Could you check a few things on this model? Use its own coordinates, in mm. A direction names the side the tool comes from. Round coordinates to 2 decimals unless told otherwise and drop trailing zeros. Loops run counter-clockwise (first coordinate to the right, second up) from the corner with the lowest first, then second, coordinate; pieces in that order, holes last. Notation, with made-up numbers: M -23.5,81 L -2.5,81 A19 ccw -2.5,94 Z; hole C 4,6 d1. An arc over 180 degrees is marked long. One line per item, written item: value. Start each with the question number.
Q1. Imagine slicing it at C-C (y = -10). Please give me the cut outline in (x, z) (3 decimals).
Q2. Which directions (+Z, -Z, +X, -X, +Y, -Y) give clear straight access to the entire face, cutting with the end or side of a thin tool? Please do faces 1 (the face through (4.639, -1.331, 5.637)), 2 (the face through (6.05, -1, 0)), 3 (the face through (-4.639, -1.331, -5.637)), 4 (the face through (-5, -2.7, 6)), 5 (the face through (-6.4, 0, 0)).
Q3. Imagine slicing it at D-D (x = 9.5). Please give me the cut outline in (y, z) (3 decimals).
Q4. Imagine slicing it at B-B (z = 0). Please give me the cut outline in (x, y).
Q5. Thinking about a two-plate mould opening in Y: for faces 6 (the face through (0, -23, 0)), 7 (the face through (10.8, -11, 0)), 8 (the face through (4.68, -1.33, -5.6)), which applies, released by +Y, released by -Y, zero draft, split by the parting line, or undercut?
Q6. I'm going to push flat-ended pins straight in: pin 1 Ø6 at (x, y) = (1.5, 3) entering from -Z; pin 2 Ø1.5 at (y, z) = (10, -3.5) entering from -X; pin 3 Ø6 at (y, z) = (-15, -3.5) entering from -X. Where does each tip first touch, or does it pass through?
Q7. Please list where these lines run through material, in increasing order: line 1 along Y through (x, z) = (6.75, 1.75); line 2 along Z through (x, y) = (0, -0.5); line 3 along X through (y, z) = (-5, -2.5).
Q8. Imagine slicing it at A-A (x = 0). Please give me the cut outline in (y, z).
Autodesk Inventor part; units mm, degrees
ref_plane "YZ Plane" through (0, 0, 0) normal (1, 0, 0) x (0, 1, 0)
ref_plane "XZ Plane" through (0, 0, 0) normal (0, 1, 0) x (-1, 0, 0)
ref_plane "XY Plane" through (0, 0, 0) normal (0, 0, 1) x (1, 0, 0)
sketch "Sketch1" plane through (0, 0, 0) normal (0, 1, 0) x (-1, 0, 0)
  circle A0 centre (0, 0) radius 7.9
  dimension "d0" = 15.8
extrude "Extrusion1" add sketch "Sketch1" along normal blind 18.9
sketch "Sketch2" plane through (0, 18.9, 0) normal (0, 1, 0) x (1, 0, 0)
  circle A0 centre (0, 0) radius 8.8
  dimension "d3" = 17.6
extrude "Extrusion2" add sketch "Sketch2" along normal blind 1.8
chamfer "Chamfer1" distance 1.5 angle 45 1 edges at (-8.8, 20.7, 0)
sketch "Sketch3" plane through (0, 0, 0) normal (0, -1, 0) x (1, 0, 0)
  line L0 (6.05, 6.7) -> (-6.05, 6.7)
  line L1 (-6.05, 6.7) -> (-6.05, -6.7)
  line L2 (-6.05, -6.7) -> (6.05, -6.7)
  line L3 (6.05, -6.7) -> (6.05, 6.7)
  line L4 (6.05, 6.7) -> (-6.05, -6.7) construction
  line L5 (-6.05, 6.7) -> (6.05, -6.7) construction
  point P0 (0, 0)
  dimension "d9" = 12.1
  dimension "d10" = 13.4
extrude "Extrusion3" add sketch "Sketch3" along normal blind 23
sketch "Sketch4" plane through (0, -23, 0) normal (0, -1, 0) x (1, 0, 0)
  line L0 (6.05, -6.7) -> (6.05, 6.7)
  line L1 (10.8, 4.525) -> (1.3, 4.525)
  line L2 (1.3, 4.525) -> (1.3, -4.525)
  line L3 (1.3, -4.525) -> (10.8, -4.525)
  line L4 (10.8, -4.525) -> (10.8, 4.525)
  line L5 (6.05, 5.0801) -> (6.05, -5.0801)
  line L6 (10.8, 4.525) -> (1.3, -4.525) construction
  line L7 (1.3, 4.525) -> (10.8, -4.525) construction
  point P0 (0, 0)
  point P1 (6.05, 0)
  dimension "d13" = 9.5
  dimension "d14" = 9.05
extrude "Extrusion4" add sketch "Sketch4" against normal blind 20.3
sketch "Sketch5" plane through (10.8, -23, 4.525) normal (1, 0, 0) x (0, 0, -1)
  line L0 (9.05, 0) -> (0, 0)
  line L1 (9.05, 4.67) -> (0, 4.67)
  line L2 (0, 4.67) -> (9.05, 4.67)
  line L3 (9.05, 4.67) -> (9.05, 0)
  line L4 (9.05, 0) -> (0, 0)
  line L5 (0, 0) -> (0, 4.67)
  point P0 (4.525, 23)
  point P1 (9.05, 4.67)
  dimension "d17" = 4.67
extrude "Extrusion5" cut sketch "Sketch5" against normal up to surface (4.75 mm away)
sketch "Sketch6" plane through (0, 0, 0) normal (0, 1, 0) x (1, 0, 0)
  circle A0 centre (0, 0) radius 7.3
  circle A1 centre (0, 0) radius 8.35
  line L0 (6.05, -6.7) -> (4.1857, -6.7)
  line L1 (-4.1857, -6.7) -> (4.1857, -6.7)
  line L2 (-4.1857, -6.7) -> (-6.05, -6.7)
  line L3 (6.05, -6.7) -> (-6.05, -6.7)
  line L4 (6.05, -4.525) -> (6.05, 4.525)
  line L5 (6.05, -4.525) -> (6.05, 4.525)
  line L6 (6.05, 6.7) -> (6.05, -6.7)
  line L7 (6.05, 6.7) -> (6.05, 5.0801)
  line L8 (6.05, -5.0801) -> (6.05, 5.0801)
  line L9 (6.05, -5.0801) -> (6.05, -6.7)
  line L10 (-6.05, 6.7) -> (-4.1857, 6.7)
  line L11 (4.1857, 6.7) -> (-4.1857, 6.7)
  line L12 (4.1857, 6.7) -> (6.05, 6.7)
  line L13 (-6.05, 6.7) -> (6.05, 6.7)
  line L14 (-6.05, -6.7) -> (-6.05, -5.0801)
  line L15 (-6.05, 5.0801) -> (-6.05, -5.0801)
  line L16 (-6.05, 5.0801) -> (-6.05, 6.7)
  line L17 (-6.05, -6.7) -> (-6.05, 6.7)
  point P0 (6.05, -5.755)
  point P1 (6.05, 5.755)
  point P2 (4.9832, 6.7)
  point P3 (-4.9832, 6.7)
  point P4 (-6.05, 5.755)
  point P5 (-6.05, -5.755)
  point P6 (-4.9832, -6.7)
  point P7 (4.9832, -6.7)
  dimension "d20" = 16.7
extrude "Extrusion6" cut sketch "Sketch6" against normal up to surface (2.7 mm away) contours A0 L4 L6 A1 | A0 L11 L12 A1 L6 L4 | L4 L6 A1 L0 L1 A0 | A0 L11 L10 A1 L12 | L1 L0 A1 L2 A0 | A0 L15 L16 A1 L10 L11 | L1 L2 A1 L14 L15 A0 | A0 L15 L14 A1 L16 | L12 L6 A1 | A1 L6 L0 | A1 L16 L10 | L2 L14 A1
properties part number "LEDpower_switch"
Report:
1. outline: M -6.05,-6.7 L 6.05,-6.7 L 6.05,-4.525 L 10.8,-4.525 L 10.8,4.525 L 6.05,4.525 L 6.05,6.7 L -6.05,6.7 Z
2. face 1: +Z, +X
2. face 2: +Z, -Z, +X
2. face 3: -Z, -X
2. face 4: +Z, -X
2. face 5: none
3. outline: M -18.33,-4.525 L -2.7,-4.525 L -2.7,4.525 L -18.33,4.525 Z
4. outline: M -8.8,18.9 L -7.9,18.9 L -7.9,0 L -6.05,0 L -6.05,-23 L 6.05,-23 L 6.05,-18.33 L 10.8,-18.33 L 10.8,-2.7 L 6.05,-2.7 L 6.05,0 L 7.9,0 L 7.9,18.9 L 8.8,18.9 L 8.8,19.2 L 7.3,20.7 L -7.3,20.7 L -8.8,19.2 Z
5. face 6: released by -Y
5. face 7: zero draft
5. face 8: undercut
6. pin 1: stops at z = -7.9
6. pin 2: stops at x = -7.41
6. pin 3: stops at x = -6.05
7. line 1: y = -18.33 to -2.7, 0 to 20.7
7. line 2: z = -6.7 to 6.7
7. line 3: x = -6.05 to 10.8
8. outline: M -23,-6.7 L 0,-6.7 L 0,-7.9 L 18.9,-7.9 L 18.9,-8.8 L 19.2,-8.8 L 20.7,-7.3 L 20.7,7.3 L 19.2,8.8 L 18.9,8.8 L 18.9,7.9 L 0,7.9 L 0,6.7 L -23,6.7 Z
